For this review, take the finished solid that the model builds, in its own axes (mm). Face numbers are marked on the shaded views. A direction names the side the tool comes from. Round coordinates to 2 decimals unless told otherwise and drop trailing zeros. Order: outer loops, then holes, each group sorted by start corner. A loop starts at its lowest first (then second) coordinate and runs counter-clockwise, first axis right, second up. Notation, with made-up numbers: (-38, 27.5) -> (20, 27.5) arc R16 ccw to (20, 38.5) -> close; hole circle Ø1 at (56, 80). An arc over 180 degrees is marked (long way). Use a Markdown table: item, result. Add a question column.
1) Consider section B-B (y = 5). State the section outline as (x, z) points.
2) Wall thickness on line 1 along Y through (x, z) = (0, 4) (3 decimals); line 2 along Z through (x, y) = (-29.5, 2.5); line 3 along X through (y, z) = (-13.5, 33.5): over which ranges is each line inside the solid? List them lowest first. Write a range as [from, to].
3) Clearance check with flat-ended pins moving along their axes: P1, Ø12, axis at y = 16, z = 19.5, coming from the -X side; P2, Ø5.5, axis at x = 30.47, y = 0.95, coming from the +Z side; P3, Ø1, axis at y = -23, z = 7.5, coming from the +X side. State where each tip first meets the part, or that it passes through.
4) Consider section A-A (x = 0). State the section outline as (y, z) points (1 decimal).
5) Draft analysis for pull direction Y (two halves, no side actions). For the marked faces 3, 4 and 5, state which applies: pulls with the +Y half, pulls with the -Y half, needs draft (parallel to the pull), parting line crosses it, or undercut.
6) Consider section C-C (z = 26). State the section outline as (x, y) points (1 decimal), plus the area to 3 significant figures.
7) Machinability: for the marked faces 1 and 2, which of the approach directions +Z, -Z, +X, -X, +Y, -Y give a long, thin tool a straight path to every point of the face, cutting with its end or side? Answer none if there is none.
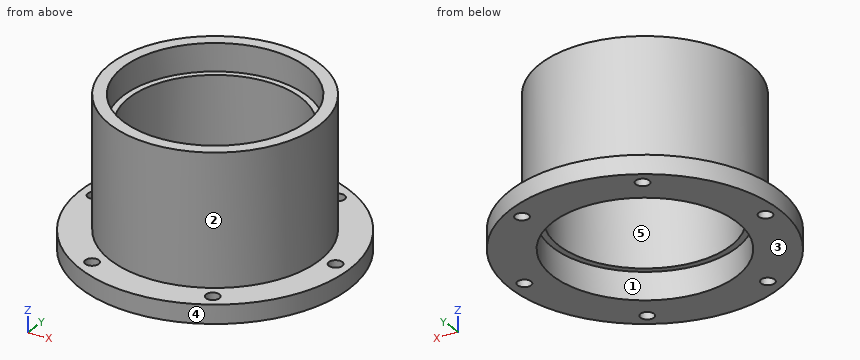
```python
from build123d import *

# Parameters (mm, degrees)
F0_R     = 34.29
F1_DEPTH = 4.7752
F2_R     = 26.67
F3_DEPTH = 33.3248
F4_R     = 21.9075
F5_DEPTH = 38.101
F6_R     = 23.495
F7_DEPTH = 7.0104
F8_R     = 23.495
F9_DEPTH = 7.0104
F11_D    = 3.4544


with BuildPart() as f1:
    # F0 (on Top) → F1 (new body)
    with BuildSketch(Plane.XY):
        Circle(F0_R)
    extrude(amount=F1_DEPTH)

    # F2 (on face) → F3 (join)
    with BuildSketch(Plane.XY.offset(4.7752)):
        Circle(F2_R)
    extrude(amount=F3_DEPTH)

    # F4 (on face) → F5 (cut, through all)
    with BuildSketch(Plane.XY.offset(38.1)):
        Circle(F4_R)
    extrude(amount=-F5_DEPTH, mode=Mode.SUBTRACT)

    # F6 (on face) → F7 (cut)
    with BuildSketch(Plane.XY.offset(38.1)):
        Circle(F6_R)
    extrude(amount=-F7_DEPTH, mode=Mode.SUBTRACT)

    # F8 (on face) → F9 (cut)
    with BuildSketch(Plane(origin=(0, 0, 0), x_dir=(1, 0, 0), z_dir=(0, 0, -1))):
        Circle(F8_R)
    extrude(amount=-F9_DEPTH, mode=Mode.SUBTRACT)

    # F11 (through all)
    with Locations(Plane(origin=(0, 0, 0), x_dir=(1, 0, 0), z_dir=(0, 0, -1))):
        with Locations((-16.052859, -25.910155), (-30.465282, 0.947107), (-14.412422, 26.857261), (16.052859, 25.910155), (30.465282, -0.947107), (14.412422, -26.857261)):
            Hole(F11_D / 2)


solid = f1.part
```
Results list:
| question | item | result |
|---|---|---|
| 1 | outline | (-33.92, 0) -> (-22.96, 0) -> (-22.96, 7.01) -> (-21.33, 7.01) -> (-21.33, 31.09) -> (-22.96, 31.09) -> (-22.96, 38.1) -> (-26.2, 38.1) -> (-26.2, 4.78) -> (-33.92, 4.78) -> close; (21.33, 7.01) -> (22.96, 7.01) -> (22.96, 0) -> (33.92, 0) -> (33.92, 4.78) -> (26.2, 4.78) -> (26.2, 38.1) -> (22.96, 38.1) -> (22.96, 31.09) -> (21.33, 31.09) -> close |
| 2 | line 1 | [-34.29, -23.495], [23.495, 34.29] |
| 2 | line 2 | [0, 4.78] |
| 2 | line 3 | [-23, -19.23], [19.23, 23] |
| 3 | P1 | x = -24.72 |
| 3 | P2 | z = 4.78 |
| 3 | P3 | x = 14.32 |
| 4 | outline | (-34.3, 0) -> (-23.5, 0) -> (-23.5, 7) -> (-21.9, 7) -> (-21.9, 31.1) -> (-23.5, 31.1) -> (-23.5, 38.1) -> (-26.7, 38.1) -> (-26.7, 4.8) -> (-34.3, 4.8) -> close; (21.9, 7) -> (23.5, 7) -> (23.5, 0) -> (34.3, 0) -> (34.3, 4.8) -> (26.7, 4.8) -> (26.7, 38.1) -> (23.5, 38.1) -> (23.5, 31.1) -> (21.9, 31.1) -> close |
| 5 | face 3 | needs draft |
| 5 | face 4 | parting line crosses it |
| 5 | face 5 | undercut |
| 6 | outline | circle Ø53.3 at (0, 0); hole circle Ø43.8 at (0, 0) |
| 6 | area | 727 mm2 |
| 7 | face 1 | -Z |
| 7 | face 2 | +Z |
